```python
from build123d import *

# Parameters (mm, degrees)
POCKET_DEPTH      = 215.522719
POCKET_DEPTH_BACK = 215.522719


with BuildPart() as part:
    # Sketch001 → Revolution (revolve)
    with BuildSketch(Plane.XZ):
        Polygon((0, 38), (0.55, 30), (0.55, 0), (0, 0), align=None)
    revolution = revolve(axis=Axis((0, 0, 0), (1, 0, 0)))

    # Mirrored: Revolution across Sketch001 V_Axis
    add(revolution.mirror(Plane(origin=(0, 0, 0), x_dir=(0, -1, 0), z_dir=(1, 0, 0))))

    # Sketch002 → Pocket (cut, two sides)
    with BuildSketch(Plane.YZ) as pocket_sk:
        with BuildLine():
            Line((3, 12.340583), (3, 16.3))
            Line((3, 16.3), (0, 16.3))
            Line((0, 16.3), (0, -12.7))
            ThreePointArc((0, -12.7), (12.609826, -1.510727), (3, 12.340583))
        make_face()
    pocket = extrude(amount=-POCKET_DEPTH, mode=Mode.SUBTRACT) + extrude(pocket_sk.sketch, amount=POCKET_DEPTH_BACK, mode=Mode.SUBTRACT)

    # Mirrored001: Pocket across Sketch002 V_Axis
    add(pocket.mirror(Plane(origin=(0, 0, 0), x_dir=(1, 0, 0), z_dir=(0, 1, 0))), mode=Mode.SUBTRACT)


solid = part.part
```
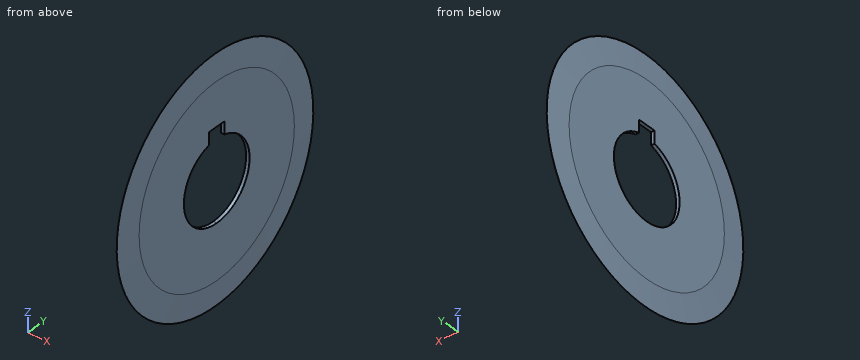
Design review of the part built by this model. Coordinates are the model's own, in mm. Coordinates: 2 decimals unless noted, no trailing zeros. Order: outer loops, then holes, each group sorted by start corner. A loop starts at its lowest first (then second) coordinate and runs counter-clockwise, first axis right, second up.
1) Take a section at B-B, the plane x = -0.3. Give the boundary of the cut face in (y, z).
2) Wall thickness on line 1 along X through (y, z) = (-0.5, -32.5); line 2 along X through (y, z) = (-2, 33.5): over which ranges is each line inside the solid? List them lowest first.
3) Take a section at A-A, the plane z = 0. Give the boundary of the cut face in (x, y), and give its area (3 significant figures).
Returned:
1. outline: circle Ø67.27 at (0, 0); hole (-3, 12.34) arc R12.7 ccw to (0, -12.7) arc R12.7 ccw to (3, 12.34) - (3, 16.3) - (-3, 16.3) - close
2. line 1: x = -0.38 to 0.38
2. line 2: x = -0.31 to 0.31
3. outline: (-0.55, -30) - (0, -38) - (0.55, -30) - (0.55, -12.7) - (-0.55, -12.7) - close; (-0.55, 12.7) - (0.55, 12.7) - (0.55, 30) - (0, 38) - (-0.55, 30) - close
3. area: 46.9 mm2
